Autodesk Inventor part; units mm, degrees
ref_plane "YZ Plane" through (0, 0, 0) normal (1, 0, 0) x (0, 1, 0)
ref_plane "XZ Plane" through (0, 0, 0) normal (0, 1, 0) x (-1, 0, 0)
ref_plane "XY Plane" through (0, 0, 0) normal (0, 0, 1) x (1, 0, 0)
sketch "Sketch1" plane through (0, 0, 0) normal (0, 0, 1) x (1, 0, 0)
  circle A0 centre (0, 0) radius 80
  circle A1 centre (0, 0) radius 225
  dimension "d0" = 160
  dimension "d1" = 450
extrude "Extrusion1" add sketch "Sketch1" along normal blind 5
sketch "Sketch2" plane through (0, 0, 5) normal (0, 0, 1) x (1, 0, 0)
  line L0 (-205, 0) -> (-100, 0) construction
  point P0 (0, 0)
  point P1 (-102.5, -177.5352)
  point P2 (-50, -86.6025)
  point P3 (102.5, -177.5352)
  point P4 (50, -86.6025)
  point P5 (205, 0)
  point P6 (100, 0)
  point P7 (102.5, 177.5352)
  point P8 (50, 86.6025)
  point P9 (-102.5, 177.5352)
  point P10 (-50, 86.6025)
  dimension "d4" = 100
  dimension "d5" = 205
  dimension "d8" = 360
hole "Hole1" at (-205, 0, 5) at (-100, 0, 5) at (-102.5, -177.5352, 5) at (-50, -86.6025, 5) at (102.5, -177.5352, 5) at (50, -86.6025, 5) at (205, 0, 5) at (100, 0, 5) at (102.5, 177.5352, 5) at (50, 86.6025, 5) at (-102.5, 177.5352, 5) at (-50, 86.6025, 5) direction (0, 0, -1) diameter 4.5 depth 8 tip angle 118
sketch "Sketch3" plane through (0, 0, 5) normal (0, 0, 1) x (1, 0, 0)
  line L0 (-137.5, -137.5) -> (137.5, -137.5) construction
  line L1 (137.5, -137.5) -> (137.5, 137.5) construction
  line L2 (137.5, 137.5) -> (-137.5, 137.5) construction
  line L3 (-137.5, 137.5) -> (-137.5, -137.5) construction
  line L4 (-137.5, -137.5) -> (137.5, 137.5) construction
  line L5 (137.5, -137.5) -> (-137.5, 137.5) construction
  point P0 (0, 0)
  dimension "d17" = 275
  dimension "d18" = 275
hole "Hole2" at (-137.5, 137.5, 5) at (137.5, -137.5, 5) at (-137.5, -137.5, 5) at (137.5, 137.5, 5) direction (0, 0, -1) diameter 5.5 depth 8 tip angle 118
sketch "Sketch4" plane through (0, 0, 5) normal (0, 0, 1) x (1, 0, 0)
  line L0 (0, 0) -> (193.1852, 51.7638) construction
  line L1 (0, 0) -> (-138.753, 0) construction
  point P0 (0, -100)
  dimension "d26" = 100
  dimension "d38" = 200
  dimension "d39" = 165
hole "Hole3" at (0, -100, 5) at (193.1852, 51.7638, 5) direction (0, 0, -1) diameter 12 depth 8 tip angle 118
properties part number "Primary" material "Polycarbonate, Clear"
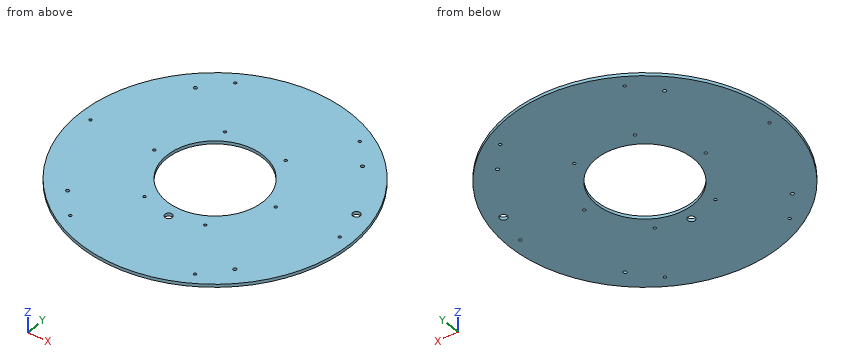
Geometry: final body of the model. Coordinates: model frame, mm. Coordinates: 2 decimals unless noted, no trailing zeros. Order: outer loops, then holes, each group sorted by start corner. A loop starts at its lowest first (then second) coordinate and runs counter-clockwise, first axis right, second up.
Item 1: Section query B-B (y = -44.5). Output: boundary loops of the cut face in (x, z), then the cut area to 3 significant figures.
Answer:
outline: (-220.56, 0) - (-66.48, 0) - (-66.48, 5) - (-220.56, 5) - close; (66.48, 0) - (220.56, 0) - (220.56, 5) - (66.48, 5) - close
area: 1,540 mm2
Item 2: Contact query for flat-ended pins moving along their axis: P1, Ø7, axis at x = 50, y = 86.6, coming from the -Z side; P2, Ø1, axis at x = 117, z = 3.5, coming from the -Y side. Output: stop coordinate, or through.
Answer:
P1: stops at z = 0
P2: stops at y = -192.49
Item 3: Material intervals for line 1 along Y through (x, z) = (0, 3.6); line 2 along Y through (x, z) = (52, 4.4); line 3 along X through (y, z) = (-135, 0.35), sorted ascending.
Answer:
line 1: y = -225 to -106, -94 to -80, 80 to 225
line 2: y = -218.91 to -87.63, -85.57 to -60.79, 60.79 to 85.57, 87.63 to 218.91
line 3: x = -180 to -138.65, -136.35 to 136.35, 138.65 to 180
Item 4: Section query D-D (x = -146.5). Output: boundary loops of the cut face in (y, z).
Answer:
outline: (-170.77, 0) - (170.77, 0) - (170.77, 5) - (-170.77, 5) - close
Item 5: Section query A-A (x = -22). Output: boundary loops of the cut face in (y, z).
Answer:
outline: (-223.92, 0) - (-76.92, 0) - (-76.92, 5) - (-223.92, 5) - close; (76.92, 0) - (223.92, 0) - (223.92, 5) - (76.92, 5) - close
Item 6: Section query C-C (z = 0.75). State how many separate pieces and enclosed holes the cut face has, then the cut area to 3 significant figures.
Answer:
separate pieces: 1
enclosed holes: 19
area: 138,000 mm2
